from build123d import *

# Parameters (mm, degrees)
SKETCH_W     = 48
SKETCH_H     = 20
PAD_DEPTH    = 1
PAD001_DEPTH = 44
POCKET_DEPTH = 20.001


with BuildPart() as part:
    # Sketch → Pad (new body)
    with BuildSketch(Plane.XY):
        Rectangle(SKETCH_W, SKETCH_H)
    extrude(amount=PAD_DEPTH)

    # Sketch001 → Pad001 (new body)
    with BuildSketch(Plane.XY.offset(1)):
        Polygon((-16, 10), (-16, -10), (19, -10), (19, -9), (-15, -9), (-15, -0.5), (19, -0.5), (19, 0.5), (-15, 0.5), (-15, 9), (19, 9), (19, 10), align=None)
    extrude(amount=PAD001_DEPTH)

    # Sketch002 → Pocket (cut, through all)
    with BuildSketch(Plane.XZ.offset(10)):
        Polygon((19, 1), (-15, 43), (-15, 46), (20, 46), (20, 1), align=None)
    extrude(amount=-POCKET_DEPTH, mode=Mode.SUBTRACT)


solid = part.part
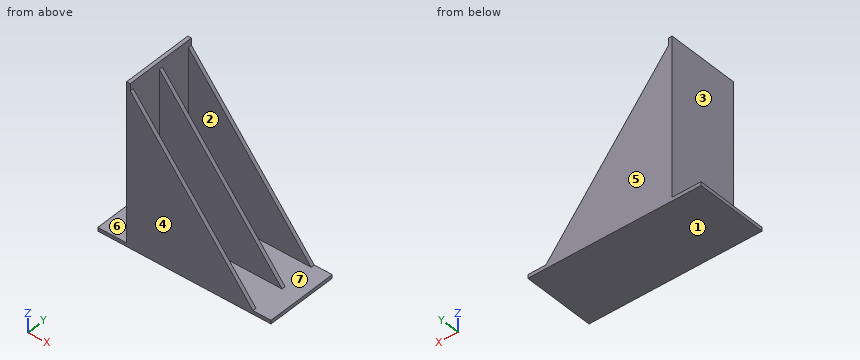
Verification items for the finished model (mm, model axes). Face numbers are marked on the shaded views. A direction names the side the tool comes from. Give positions to 0.01 mm unless a question says otherwise; leave off trailing zeros. Order: outer loops, then holes, each group sorted by start corner. A loop starts at its lowest first (then second) coordinate and runs counter-clockwise, first axis right, second up. Notation, with made-up numbers: M 15,28.25 L 34,28.25 A35 cw 34,67.25 Z; hole C 36.5,26 d4. An arc over 180 degrees is marked long. Use one line per item in the form item = value. Start each with the question number.
Q1. Scan lines: line 1 along Y through (x, z) = (-8.5, 21.5); line 2 along X through (y, z) = (-5.5, 35); line 3 along Z through (x, y) = (13, 6.25). Record each from-to range of solid material in increasing order. Write a range as [from, to].
Q2. Go/stop test with flat-tipped pins: pin 1 Ø4 at (y, z) = (-7.5, 20) entering from +X; pin 2 Ø6 at (x, y) = (6, -5.5) entering from +Z; pin 3 Ø10 at (y, z) = (-0.5, 35.5) entering from +X. Record where each tip stops, or that it passes through.
Q3. Section check D-D (x = -17). Enter the section's corners in (y, z).
Q4. Section check B-B (z = 10.5). Enter the section's corners in (x, y), then the cut area to 3 significant figures.
Q5. Section check C-C (x = -5.5). Enter the section's corners in (y, z).
Q6. Section check A-A (y = 8). Enter the section's corners in (x, z).
Q7. Access from +Z, -Z, +X, -X, +Y, -Y to the whole of each face (thin tool, end or side, straight path). Record for the marked faces 1, 2 and 3.
Q8. Mould release check, pull along Y, two halves, no side actions. Record for the marked faces 4, 5, 6 and 7: +Y half, -Y half, draft (parallel to the pull), parting line (faces both ways), or undercut.
Evaluation:
q1.line_1 = [-10, -9], [-0.5, 0.5], [9, 10]
q1.line_2 = [-16, -15]
q1.line_3 = [0, 1]
q2.pin_1 = 4.69
q2.pin_2 = 1
q2.pin_3 = -4.88
q3.outline = M -10,0 L 10,0 L 10,1 L -10,1 Z
q4.outline = M -16,-10 L 11.31,-10 L 11.31,-9 L -15,-9 L -15,-0.5 L 11.31,-0.5 L 11.31,0.5 L -15,0.5 L -15,9 L 11.31,9 L 11.31,10 L -16,10 Z
q4.area = 98.9 mm2
q5.outline = M -10,0 L 10,0 L 10,31.26 L 9,31.26 L 9,1 L 0.5,1 L 0.5,31.26 L -0.5,31.26 L -0.5,1 L -9,1 L -9,31.26 L -10,31.26 Z
q6.outline = M -24,0 L 24,0 L 24,1 L -15,1 L -15,45 L -16,45 L -16,1 L -24,1 Z
q7.face_1 = -Z, +X, -X, +Y, -Y
q7.face_2 = +Z, +X
q7.face_3 = +Z, -X, +Y, -Y
q8.face_4 = -Y half
q8.face_5 = +Y half
q8.face_6 = draft
q8.face_7 = undercut
